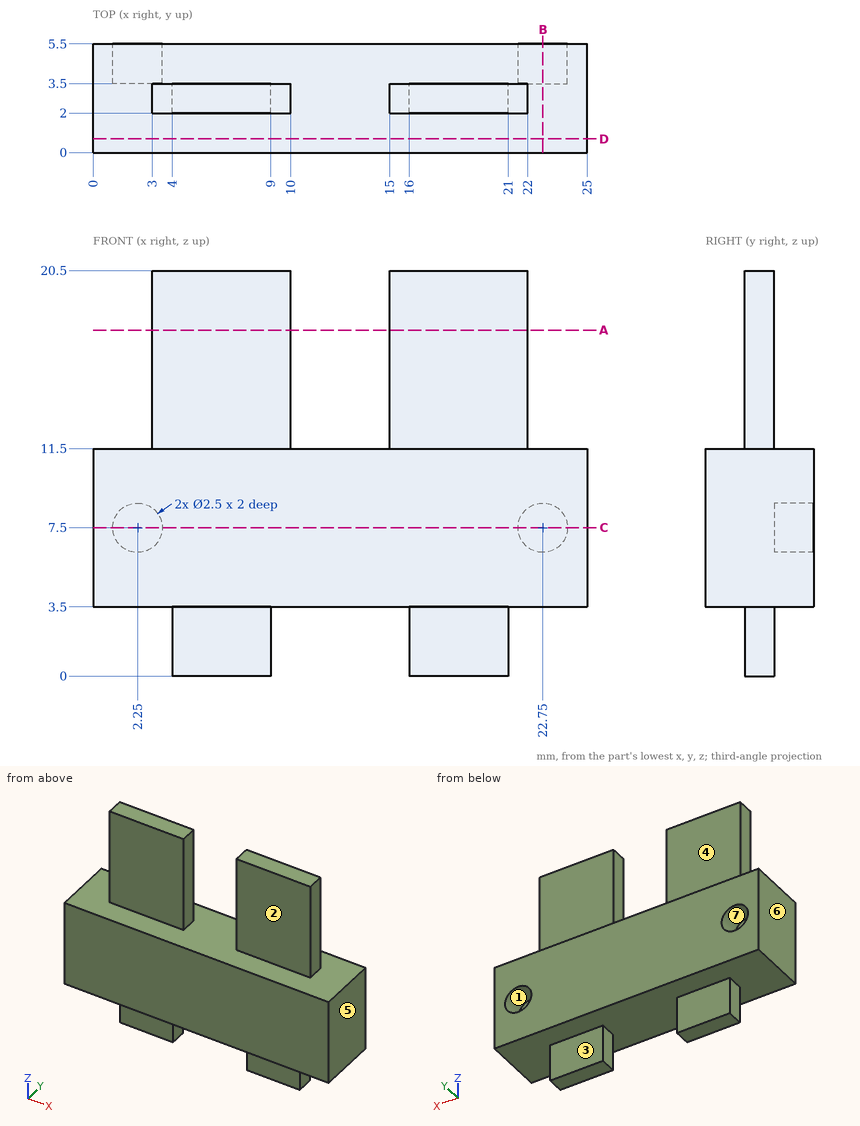
Geometry: see drawing. Coordinates: mm, zero at the bounding-box minimum. A direction names the side the tool comes from. Give positions to 0.01 mm unless a question says otherwise; leave off trailing zeros. Loops run counter-clockwise (first coordinate to the right, second up) from the corner with the lowest first, then second, coordinate; pieces in that order, holes last. Notation, with made-up numbers: (81.5, 59.5) - (114.5, 59.5) arc R20 ccw to (114.5, 90.5) - close; hole circle Ø10 at (8.25, 5.5). An arc over 180 degrees is marked (long way). Answer as CSV lines item,"result". Start each with the question number.
1. Section B-B, the plane x = 22.75. Return loops of the section in (y, z), plus the area to 3 significant figures.
2. Section D-D, the plane y = 0.7. Return loops of the section in (x, z), plus the area to 3 significant figures.
3. Section C-C, the plane z = 7.5. Return loops of the section in (x, y).
4. Pin query (flat end, axial travel): P1, Ø3.5, axis at x = 18, z = 14.5, coming from the +Y side; P2, Ø1.2, axis at y = 3, z = 2.5, coming from the +X side; P3, Ø3.5, axis at x = 17.5, z = 15, coming from the -Y side; P4, Ø1, axis at y = 4.5, z = 14.5, coming from the -X side. Return the tip coordinate at first contact, or that it passes through.
5. Section A-A, the plane z = 17.5. Return loops of the section in (x, y).
6. Draft query along X for the marked faces 4, 5, 6 and 7. Return one class per face: released by +X, released by -X, zero draft, split by the parting line, or undercut.
7. Reachability of the marked faces 1, 2 and 3 from +Z, -Z, +X, -X, +Y, -Y: full face, straight path, thin tool, end or side. Return the list, or none.
8. Ray query, L1, parallel to X at y = 4.3, z = 7.5; L2, parallel to Z at x = 22.75, y = 4; L3, parallel to X at y = 2.7, z = 12. Return the intervals inside material, ascending.
Answers:
1,outline,"(0, 3.5) - (5.5, 3.5) - (5.5, 6.25) - (3.5, 6.25) - (3.5, 8.75) - (5.5, 8.75) - (5.5, 11.5) - (0, 11.5) - close"
1,area,"39.0 mm2"
2,outline,"(0, 3.5) - (25, 3.5) - (25, 11.5) - (0, 11.5) - close"
2,area,"200 mm2"
3,outline,"(0, 0) - (25, 0) - (25, 5.5) - (24, 5.5) - (24, 3.5) - (21.5, 3.5) - (21.5, 5.5) - (3.5, 5.5) - (3.5, 3.5) - (1, 3.5) - (1, 5.5) - (0, 5.5) - close"
4,P1,"stops at y = 3.5"
4,P2,"stops at x = 21"
4,P3,"stops at y = 2"
4,P4,"passes through"
5,outline,"(3, 2) - (10, 2) - (10, 3.5) - (3, 3.5) - close; (15, 2) - (22, 2) - (22, 3.5) - (15, 3.5) - close"
6,face 4,"zero draft"
6,face 5,"released by +X"
6,face 6,"released by -X"
6,face 7,"undercut"
7,face 1,"+Y"
7,face 2,"+Z, +X, -X, -Y"
7,face 3,"-Z, +X, -X, +Y"
8,L1,"x = 0 to 1, 3.5 to 21.5, 24 to 25"
8,L2,"z = 3.5 to 6.25, 8.75 to 11.5"
8,L3,"x = 3 to 10, 15 to 22"
